```python
from build123d import *

# Parameters (mm, degrees)
SKETCH1_W           = 145.885353282
SKETCH1_H           = 101.6
BOSS_EXTRUDE1_DEPTH = 3.2004
SKETCH4_W           = 57.100000132
SKETCH4_H           = 31.75
CUT_EXTRUDE1_DEPTH  = 3.2004
SKETCH5_R           = 2.159
CUT_EXTRUDE2_DEPTH  = 3.2004
SKETCH7_R           = 1.1303
CUT_EXTRUDE3_DEPTH  = 3.2004
SKETCH9_W           = 7.62
SKETCH9_H           = 3.175
CUT_EXTRUDE5_DEPTH  = 3.2004
SKETCH10_R          = 0.59563
CUT_EXTRUDE6_DEPTH  = 3.2004
FILLET1_R           = 0.762
SKETCH11_R          = 1.7272
CUT_EXTRUDE7_DEPTH  = 3.2004


with BuildPart() as part:
    # Sketch1 → Boss-Extrude1 (new body)
    with BuildSketch(Plane.XY):
        with Locations((72.942676641, 50.8)):
            Rectangle(SKETCH1_W, SKETCH1_H)
    extrude(amount=BOSS_EXTRUDE1_DEPTH)

    # Sketch4 → Cut-Extrude1 (cut)
    with BuildSketch(Plane.XY.offset(3.2004)):
        with Locations((56.982760066, 15.875)):
            Rectangle(SKETCH4_W, SKETCH4_H)
    extrude(amount=-CUT_EXTRUDE1_DEPTH, mode=Mode.SUBTRACT)

    # Sketch5 → Cut-Extrude2 (cut)
    with BuildSketch(Plane.XY.offset(3.2004)):
        with Locations((141.376853282, 82.55)):
            Circle(SKETCH5_R)
        with Locations((141.376853282, 19.05)):
            Circle(SKETCH5_R)
        with Locations((4.5085, 19.05)):
            Circle(SKETCH5_R)
        with Locations((4.5085, 82.55)):
            Circle(SKETCH5_R)
        with Locations((21.31994339, 79.375)):
            Circle(SKETCH5_R)
        with Locations((21.31994339, 22.225)):
            Circle(SKETCH5_R)
        with Locations((122.472903282, 79.375)):
            Circle(SKETCH5_R)
        with Locations((122.472903282, 22.225)):
            Circle(SKETCH5_R)
    extrude(amount=-CUT_EXTRUDE2_DEPTH, mode=Mode.SUBTRACT)

    # Sketch7 → Cut-Extrude3 (cut)
    with BuildSketch(Plane(origin=(0, 0, 0), x_dir=(-1, 0, 0), z_dir=(0, 0, -1))):
        with Locations((-40.438191852, 91.294483225)):
            Circle(SKETCH7_R)
        with Locations((-40.438191852, 70.974483225)):
            Circle(SKETCH7_R)
        with Locations((-65.838191852, 70.974483225)):
            Circle(SKETCH7_R)
        with Locations((-65.838191852, 91.294483225)):
            Circle(SKETCH7_R)
        with Locations((-72.507486221, 61.720086416)):
            Circle(SKETCH7_R)
        with Locations((-72.507486221, 41.400086416)):
            Circle(SKETCH7_R)
        with Locations((-97.907486221, 41.400086416)):
            Circle(SKETCH7_R)
        with Locations((-97.907486221, 61.720086416)):
            Circle(SKETCH7_R)
    extrude(amount=-CUT_EXTRUDE3_DEPTH, mode=Mode.SUBTRACT)

    # Sketch9 → Cut-Extrude5 (cut)
    with BuildSketch(Plane.XY.offset(3.2004)):
        with Locations((110.993373282, 100.0125)):
            Rectangle(SKETCH9_W, SKETCH9_H)
        with Locations((110.993373282, 1.5875)):
            Rectangle(SKETCH9_W, SKETCH9_H)
        with Locations((24.62276, 1.5875)):
            Rectangle(SKETCH9_W, SKETCH9_H)
    extrude(amount=-CUT_EXTRUDE5_DEPTH, mode=Mode.SUBTRACT)

    # Sketch10 → Cut-Extrude6 (cut)
    with BuildSketch(Plane.XY.offset(3.2004)):
        with Locations((98.232760132, 24.47)):
            Circle(SKETCH10_R)
        with Locations((134.232760132, 24.47)):
            Circle(SKETCH10_R)
        with Locations((98.232760132, 3.47)):
            Circle(SKETCH10_R)
        with Locations((134.232760132, 3.47)):
            Circle(SKETCH10_R)
    extrude(amount=-CUT_EXTRUDE6_DEPTH, mode=Mode.SUBTRACT)

    # Fillet1
    fillet1_edges = [part.edges().sort_by_distance(p)[0] for p in [
        (114.803373282, 101.6, 1.6002),
        (107.183373282, 101.6, 1.6002),
        (114.803373282, 0, 1.6002),
        (107.183373282, 0, 1.6002),
        (28.43276, 3.175, 1.6002),
        (20.81276, 0, 1.6002),
        (85.532760132, 0, 1.6002),
        (0, 101.6, 1.6002),
        (145.885353282, 101.6, 1.6002),
        (145.885353282, 0, 1.6002),
        (0, 0, 1.6002),
    ]]
    fillet(fillet1_edges, radius=FILLET1_R)

    # Sketch11 → Cut-Extrude7 (cut)
    with BuildSketch(Plane.XY.offset(3.2004)):
        with Locations((13.252676641, 55.5625)):
            Circle(SKETCH11_R)
        with Locations((13.252676641, 80.9625)):
            Circle(SKETCH11_R)
        with Locations((132.632676641, 55.5625)):
            Circle(SKETCH11_R)
        with Locations((132.632676641, 80.9625)):
            Circle(SKETCH11_R)
        with Locations((107.232676641, 33.3375)):
            Circle(SKETCH11_R)
        with Locations((94.532676641, 33.3375)):
            Circle(SKETCH11_R)
    extrude(amount=-CUT_EXTRUDE7_DEPTH, mode=Mode.SUBTRACT)


solid = part.part
```
Check sheet for the modelled part. Datum: model origin and axes. Units: mm. A direction names the side the tool comes from. Round coordinates to 2 decimals unless told otherwise and drop trailing zeros. Order: outer loops, then holes, each group sorted by start corner. A loop starts at its lowest first (then second) coordinate and runs counter-clockwise, first axis right, second up.
1) Section check B-B (x = 54.5). Record the boundary of the cut face in (y, z), and give its area (3 significant figures).
2) Section check A-A (y = 26.5). Record the boundary of the cut face in (x, z), and give its area (3 significant figures).
3) Section check C-C (z = 1.65). Give the number of separate pieces and of enclosed holes in the cut face, and give its area (3 significant figures).
4) Mould release check, pull along X, two halves, no side actions. Record for faces 1 (the cylindrical face through (143.37, 81.72, 1.62)), 2 (the flat face through (53, 101.6, 2)): +X half, -X half, draft (parallel to the pull), parting line (faces both ways), or undercut.
5) Scan lines: line 1 (X direction, y = 54, z = 2.5); line 2 (X direction, y = 15.5, z = 2.2); line 3 (X direction, y = 70.5, z = 0.4). Record each from-to range of solid material in increasing order.
6) Tool access check on faces 3 (the cylindrical face through (4.23, 21.19, 1.62)), 4 (the flat face through (28.433, 18, 2)). Record the directions out of +Z, -Z, +X, -X, +Y, -Y that give a thin tool (end or side, any length) a straight path to the whole face; none if there is none.
Result:
1. outline: (31.75, 0) - (101.6, 0) - (101.6, 3.2) - (31.75, 3.2) - close
1. area: 224 mm2
2. outline: (0, 0) - (28.43, 0) - (28.43, 3.2) - (0, 3.2) - close; (85.53, 0) - (145.89, 0) - (145.89, 3.2) - (85.53, 3.2) - close
2. area: 284 mm2
3. separate pieces: 1
3. enclosed holes: 26
3. area: 12,700 mm2
4. face 1: undercut
4. face 2: draft
5. line 1: x = 0 to 12.52, 13.99 to 131.9, 133.37 to 145.89
5. line 2: x = 0 to 28.43, 85.53 to 145.89
5. line 3: x = 0 to 39.41, 41.46 to 64.81, 66.86 to 145.89
6. face 3: +Z, -Z
6. face 4: +Z, -Z, -Y
